Geometry: final body of the model. Coordinates: model frame, mm. Face numbers are marked on the shaded views. A direction names the side the tool comes from. Coordinates: 2 decimals unless noted, no trailing zeros. Write each loop counter-clockwise with the first axis right and the second up, starting at its lowest first coordinate (ties: lowest second). Pieces come first, ordered by that corner, then holes. Notation, with made-up numbers: (18, 37) - (31, 37) arc R21 cw to (31, 58) - close; hole circle Ø9 at (-3, -10.75). An arc over 180 degrees is marked (long way). Answer as a JSON object with one key per item and string values. Group by question number.
Item 1: First-contact query: pin 1 Ø3 at (x, y) = (15, 18.5) entering from -Z; pin 2 Ø6 at (y, z) = (13, -10.5) entering from +X; pin 3 Ø2.5 at (x, y) = (1.5, -6.5) entering from +Z. Flat tips, straight axial feed; report the tip coordinate or a pass-through.
Item 2: Section B-B on z = -2. Return loops of the section in (x, y) (3 decimals).
Item 3: Set-up query: the marked faces 1, 2 and 3. Return all of +Z, -Z, +X, -X, +Y, -Y with unobstructed straight access to the full face (end or side cutting, diameter ignored); none if empty.
Item 4: Mould query, pull axis X, two halves, no side actions, for the marked faces 4, 5 and 6. Classes: pulls with the +X half, pulls with the -X half, needs draft (parallel to the pull), parting line crosses it, or undercut.
Item 5: Section A-A on y = -16. State how many separate pieces and enclosed holes the cut face has, and give its area (3 significant figures).
Item 6: Line query: line 1 along X through (y, z) = (-20, 48); line 2 along Z through (x, y) = (70, 7); line 3 along X through (y, z) = (10, -5). Output: solid intervals per line, ascending. Write a range as from..to.
Item 7: Section C-C on x = 144. Return loops of the section in (y, z).
```python
from build123d import *

# Parameters (mm, degrees)
F0_R     = 22.225
F1_DEPTH = 12.7
F0_R_2   = 9.525
F0_R_3   = 14.2875
F2_DEPTH = 22.225


with BuildPart() as f1:
    # F0 (on Front) → F1 (new body, symmetric)
    with BuildSketch(Plane.XZ):
        with BuildLine():
            ThreePointArc((0, -19.05), (-1.654463, -18.97802), (-3.296423, -18.762625))
            Line((-3.296423, -18.762625), (88.6968, -34.925))
            ThreePointArc((88.6968, -34.925), (103.485961, -31.639158), (115.492311, -22.399915))
            ThreePointArc((115.492311, -22.399915), (125.067877, -16.921755), (135.901052, -19.005989))
            ThreePointArc((135.901052, -19.005989), (158.328168, -19.36485), (169.6466, 0))
            ThreePointArc((169.6466, 0), (164.76473, 27.686462), (150.707944, 52.033528))
            ThreePointArc((150.707944, 52.033528), (133.25733, 59.968505), (116.123111, 51.371624))
            ThreePointArc((116.123111, 51.371624), (101.35138, 45.385387), (88.826782, 55.24305))
            ThreePointArc((88.826782, 55.24305), (89.916646, 51.503113), (90.2843, 47.625))
            ThreePointArc((90.2843, 47.625), (69.6468, 26.9875), (49.0093, 47.625))
            ThreePointArc((49.0093, 47.625), (33.876078, 27.660393), (10.350325, 19.05))
            Line((10.350325, 19.05), (25.4, 19.05))
            ThreePointArc((25.4, 19.05), (44.45, 0), (25.4, -19.05))
            Line((25.4, -19.05), (0, -19.05))
        make_face()
        with Locations((88.6968, 0)):
            Circle(F0_R, mode=Mode.SUBTRACT)
        with BuildLine():
            ThreePointArc((158.5468, 0), (147.4216, -11.1252), (136.2964, 0))
            ThreePointArc((136.2964, 0), (133.425793, 16.280022), (125.160209, 30.596433))
            ThreePointArc((125.160209, 30.596433), (126.531466, 46.269971), (142.205004, 44.898715))
            ThreePointArc((142.205004, 44.898715), (154.33433, 23.890107), (158.5468, 0))
        make_face(mode=Mode.SUBTRACT)
    extrude(amount=F1_DEPTH, both=True)

    # F0 (on Front) → F2 (join, symmetric)
    with BuildSketch(Plane.XZ):
        with BuildLine():
            Line((4.5593, 19.05), (0, 19.05))
            ThreePointArc((0, 19.05), (-18.97802, 1.654463), (-3.296423, -18.762625))
            ThreePointArc((-3.296423, -18.762625), (-1.654463, -18.97802), (0, -19.05))
            Line((0, -19.05), (25.4, -19.05))
            ThreePointArc((25.4, -19.05), (44.45, 0), (25.4, 19.05))
            Line((25.4, 19.05), (10.350325, 19.05))
            ThreePointArc((10.350325, 19.05), (7.454813, 18.955592), (4.5593, 19.05))
        make_face()
        with BuildLine():
            ThreePointArc((0, -11.0998), (-11.0998, 0), (0, 11.0998))
            Line((0, 11.0998), (25.4, 11.0998))
            ThreePointArc((25.4, 11.0998), (36.4998, 0), (25.4, -11.0998))
            Line((25.4, -11.0998), (0, -11.0998))
        make_face(mode=Mode.SUBTRACT)
        with BuildLine():
            ThreePointArc((88.826782, 55.24305), (65.768687, 67.894846), (49.0093, 47.625))
            ThreePointArc((49.0093, 47.625), (69.6468, 26.9875), (90.2843, 47.625))
            ThreePointArc((90.2843, 47.625), (89.916646, 51.503113), (88.826782, 55.24305))
        make_face()
        with Locations((69.6468, 47.625)):
            Circle(F0_R_2, mode=Mode.SUBTRACT)
        with Locations((88.6968, 0)):
            Circle(F0_R)
        with Locations((88.6968, 0)):
            Circle(F0_R_3, mode=Mode.SUBTRACT)
    extrude(amount=F2_DEPTH, both=True)


solid = f1.part
```
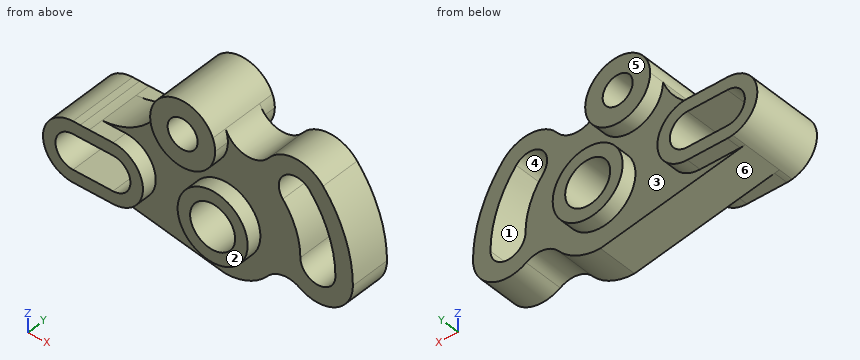
Checks:
{
 "1": {"pin 1": "z = -19.05", "pin 2": "x = 168.34", "pin 3": "z = 19.05"},
 "2": {"outline": "(-18.945, -22.225) - (-10.918, -22.225) - (-10.918, 22.225) - (-18.945, 22.225) - close; (36.318, -22.225) - (44.345, -22.225) - (44.345, -12.7) - (66.562, -12.7) - (66.562, -22.225) - (74.55, -22.225) - (74.55, 22.225) - (66.562, 22.225) - (66.562, 12.7) - (44.345, 12.7) - (44.345, 22.225) - (36.318, 22.225) - close; (102.844, -22.225) - (110.832, -22.225) - (110.832, -12.7) - (136.478, -12.7) - (136.478, 12.7) - (110.832, 12.7) - (110.832, 22.225) - (102.844, 22.225) - close; (158.366, -12.7) - (169.556, -12.7) - (169.556, 12.7) - (158.366, 12.7) - close"},
 "3": {"face 1": "+Y, -Y", "face 2": "+Z, -Z, +X, -X, -Y", "face 3": "+Y"},
 "4": {"face 4": "undercut", "face 5": "needs draft", "face 6": "pulls with the -X half"},
 "5": {"separate pieces": "3", "enclosed holes": "3", "area": "3,120 mm^2"},
 "6": {"line 1": "49.01..60.13, 79.16..90.28", "line 2": "-31.64..38.11, 57.14..68.26", "line 3": "-18.38..-9.91, 35.31..75.31, 102.08..137.48, 157.36..169.08"},
 "7": {"outline": "(-12.7, -21.96) - (12.7, -21.96) - (12.7, -10.59) - (-12.7, -10.59) - close; (-12.7, 42.67) - (12.7, 42.67) - (12.7, 57.43) - (-12.7, 57.43) - close"}
}
